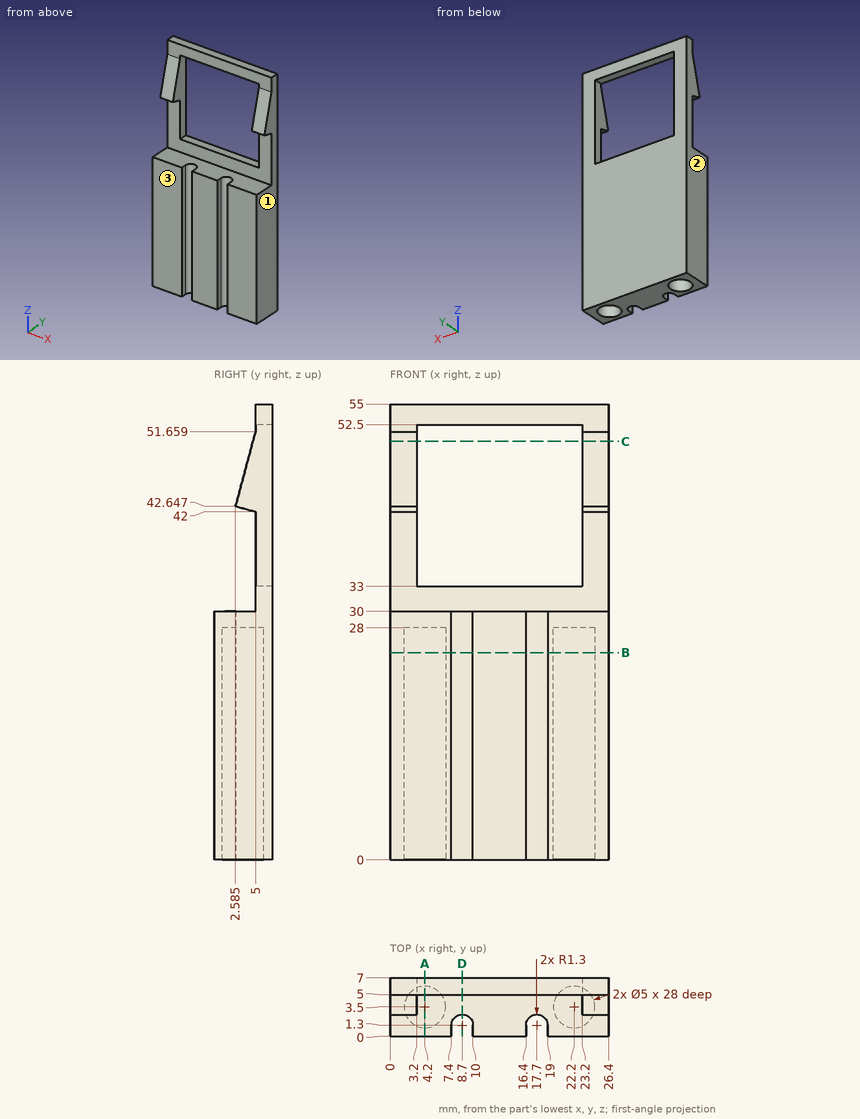
Answer from the drawing. Dimensions are ordinates in mm from the lowest x, y and z of the part. Coordinates: 2 decimals unless noted, no trailing zeros. Loops run counter-clockwise (first coordinate to the right, second up) from the corner with the lowest first, then second, coordinate; pieces in that order, holes last. Notation, with made-up numbers: (51, 17.5) - (82, 17.5) arc R15 ccw to (82, 30.5) - close; hole circle Ø6 at (-10, -35.75). An arc over 180 degrees is marked (long way). Answer in a Markdown table with one row per item.
1. Straight lines are drawn through the part: line 1 (Y direction, x = 4.2, z = 12); line 2 (X direction, y = 3.5, z = 42.5); line 3 (X direction, y = 4.75, z = 22) (1 decimal). For each, find the intervals that lie inside material, in ascending order.
Conclusion:
| item | result |
|---|---|
| line 1 | y = 0 to 1, 6 to 7 |
| line 2 | x = 0 to 3.2, 23.2 to 26.4 |
| line 3 | x = 0 to 2, 6.4 to 20, 24.4 to 26.4 |
2. Find section D-D, the plane x = 8.7. Write down the section's boundary in (y, z).
Conclusion:
| item | result |
|---|---|
| outline | (2.6, 0) - (7, 0) - (7, 33) - (5, 33) - (5, 30) - (2.6, 30) - close; (5, 52.5) - (7, 52.5) - (7, 55) - (5, 55) - close |
3. Given pin 1 (3 mm diameter, centred on x = 14, z = 14, fed in from -Y); pin 2 (3 mm diameter, centred on x = 22.2, y = 3.5, fed in from -Z); pin 3 (2.5 mm diameter, centred on x = 19, z = 53, fed in from -Y); pin 4 (9.5 mm diameter, centred on x = 10, z = 38.5, fed in from -Y), each flat-ended and moving along its own axis, determine where each tip first touches the part or whether it passes through.
Conclusion:
| item | result |
|---|---|
| pin 1 | stops at y = 0 |
| pin 2 | stops at z = 28 |
| pin 3 | stops at y = 5 |
| pin 4 | passes through |
4. Find section C-C, the plane z = 50.5. Write down the section's boundary in (x, y).
Conclusion:
| item | result |
|---|---|
| outline | (0, 4.69) - (3.2, 4.69) - (3.2, 7) - (0, 7) - close; (23.2, 4.69) - (26.4, 4.69) - (26.4, 7) - (23.2, 7) - close |
5. Determine the mould class of the marked faces 1, 2 and 3 for opening direction X: +X half, -X half, draft (parallel to the pull), parting line (faces both ways), or undercut.
Conclusion:
| item | result |
|---|---|
| face 1 | +X half |
| face 2 | -X half |
| face 3 | draft |
6. Find section A-A, the plane x = 4.2. Write down the section's boundary in (y, z).
Conclusion:
| item | result |
|---|---|
| outline | (0, 0) - (1, 0) - (1, 28) - (6, 28) - (6, 0) - (7, 0) - (7, 33) - (5, 33) - (5, 30) - (0, 30) - close; (5, 52.5) - (7, 52.5) - (7, 55) - (5, 55) - close |
7. Find section B-B, the plane z = 25. Write down the section's boundary in (x, y).
Conclusion:
| item | result |
|---|---|
| outline | (0, 0) - (7.4, 0) - (7.4, 1.3) arc R1.3 cw to (10, 1.3) - (10, 0) - (16.4, 0) - (16.4, 1.3) arc R1.3 cw to (19, 1.3) - (19, 0) - (26.4, 0) - (26.4, 7) - (0, 7) - close; hole circle Ø5 at (4.2, 3.5); hole circle Ø5 at (22.2, 3.5) |
